Here's how the part is built. I have some questions about the finished solid (model axes, mm). A direction names the side the tool comes from. Coordinates: 2 decimals unless noted, no trailing zeros. Write each loop counter-clockwise with the first axis right and the second up, starting at its lowest first coordinate (ties: lowest second). Pieces come first, ordered by that corner, then holes.
Item 1: If we section it at A-A (x = 8.5): Please give me the cut outline in (y, z), then the cut area to 3 significant figures.
Item 2: If I drill on line 1 (Z direction, x = 17.5, y = 1.5); line 2 (Z direction, x = 4, y = 8.5); line 3 (Z direction, x = 22, y = 9), over which ranges is the centre line in solid material (lowest first)?
Item 3: If we section it at B-B (z = -3.5): Please give me the cut outline in (x, y), then the cut area to 3 significant figures.
Item 4: We'd pull the mould along Z, two halves only. Please class faces 4 (the face through (8, 6, -6)), 5 (the face through (0, 6, -18)), 6 (the face through (9.5, 4.5, -30)), 7 (the face through (17, 6, -25)): +Z half, -Z half, draft (parallel to the pull), parting line (faces both ways), or undercut.
Item 5: I'm going to push flat-ended pins straight in: pin 1 Ø0.8 at (y, z) = (3.5, -24.5) entering from +X; pin 2 Ø0.8 at (y, z) = (6, -5.5) entering from -X. Where does each tip first touch, or does it pass through?
Item 6: If we section it at D-D (y = 11): Please give me the cut outline in (x, z), then the cut area to 3 significant figures.
Item 7: If we section it at C-C (x = 2.5): Please give me the cut outline in (y, z), then the cut area to 3 significant figures.
Item 8: For faces 1 (the face through (9.5, 4.5, 0)), 2 (the face through (5, 6, -24.5)), 3 (the face through (20, 6, -5.5)), which set-ups out of +Z, -Z, +X, -X, +Y, -Y let a thin tool reach every point of the face, with its end or its side?
from build123d import *

# Parameters (mm, degrees)
SKETCH_1_W          = 25
SKETCH_1_H          = 30
EXTRUDE_1_DEPTH     = 11.8
SKETCH_2_W          = 20
SKETCH_2_H          = 1
CUT_EXTRUDE_1_DEPTH = 13.5
CUT_EXTRUDE_2_DEPTH = 30


with BuildPart() as part:
    # 草图1 → 凸台-拉伸1 (new body)
    with BuildSketch(Plane(origin=(0, 0, 0), x_dir=(1, 0, 0), z_dir=(0, 1, 0))):
        with Locations((12.5, 15)):
            Rectangle(SKETCH_1_W, SKETCH_1_H)
    extrude(amount=EXTRUDE_1_DEPTH)

    # 草图2 → 切除-拉伸1 (cut)
    with BuildSketch(Plane(origin=(0, 11.8, 0), x_dir=(1, 0, 0), z_dir=(0, 1, 0))):
        with Locations((15, 24.5)):
            Rectangle(SKETCH_2_W, SKETCH_2_H)
        with Locations((10, 5.5)):
            Rectangle(SKETCH_2_W, SKETCH_2_H)
    extrude(amount=-CUT_EXTRUDE_1_DEPTH, mode=Mode.SUBTRACT)

    # 草图3 → 切除-拉伸2 (cut)
    with BuildSketch(Plane(origin=(0, 0, -30), x_dir=(-1, 0, 0), z_dir=(0, 0, -1))):
        with BuildLine():
            ThreePointArc((-9.5, 5.9), (-10.378679656, 8.021320344), (-12.5, 8.9))
            Line((-12.5, 8.9), (-12.5, 2.9))
            ThreePointArc((-12.5, 2.9), (-10.378679656, 3.778679656), (-9.5, 5.9))
        make_face()
        with BuildLine():
            Line((-12.5, 2.9), (-12.5, 8.9))
            ThreePointArc((-12.5, 8.9), (-15.5, 5.9), (-12.5, 2.9))
        make_face()
    extrude(amount=-CUT_EXTRUDE_2_DEPTH, mode=Mode.SUBTRACT)


solid = part.part
Answer list:
1. outline: (0, -30) - (11.8, -30) - (11.8, -25) - (0, -25) - close; (0, -24) - (11.8, -24) - (11.8, -6) - (0, -6) - close; (0, -5) - (11.8, -5) - (11.8, 0) - (0, 0) - close
1. area: 330 mm2
2. line 1: z = -30 to -25, -24 to -6, -5 to 0
2. line 2: z = -30 to -6, -5 to 0
2. line 3: z = -30 to -25, -24 to 0
3. outline: (0, 0) - (25, 0) - (25, 11.8) - (0, 11.8) - close; hole circle Ø6 at (12.5, 5.9)
3. area: 267 mm2
4. face 4: undercut
4. face 5: draft
4. face 6: -Z half
4. face 7: undercut
5. pin 1: stops at x = 5
5. pin 2: stops at x = 20
6. outline: (0, -30) - (25, -30) - (25, -25) - (5, -25) - (5, -24) - (25, -24) - (25, 0) - (0, 0) - (0, -5) - (20, -5) - (20, -6) - (0, -6) - close
6. area: 710 mm2
7. outline: (0, -30) - (11.8, -30) - (11.8, -6) - (0, -6) - close; (0, -5) - (11.8, -5) - (11.8, 0) - (0, 0) - close
7. area: 342 mm2
8. face 1: +Z, +X, -X, +Y, -Y
8. face 2: +X, +Y, -Y
8. face 3: -X, +Y, -Y
